CAD build for the part. Positions are in the model's coordinates, mm. A direction names the side the tool comes from. Round coordinates to 2 decimals unless told otherwise and drop trailing zeros. Order: outer loops, then holes, each group sorted by start corner. A loop starts at its lowest first (then second) coordinate and runs counter-clockwise, first axis right, second up. Notation, with made-up numbers: (-7.75, -6.75) -> (1.25, -6.75) arc R19 cw to (1.25, 29.25) -> close; hole circle Ø1 at (-25.75, -40). An arc over 180 degrees is marked (long way). Return JSON: item names as keys, results as strings. Group by question number.
Q1. Which spindle directions (+Z, -Z, +X, -X, +Y, -Y) get a long thin tool onto all of the face, cutting with end or side? Do faces 1 (the cylindrical face through (-10.67, 23.42, 31.62)), 2 (the flat face through (-4, -1, -11.1)), 3 (the flat face through (0, 13, 30.1)). Say none if no direction does.
Q2. Flat gauge pin, fed straight in: pin 1 (2.5 mm diameter, centred on x = -11, z = -34, fed in from +Y). Where does the tip first touch, or does it go through?
Q3. Cut at B-B (x = 11). Write the cut outline in (y, z), then the cut area to 3 significant figures.
Q4. Cut at D-D (z = -34.1). Write the cut outline in (x, y), then the cut area to 3 significant figures.
Q5. Probe line 1 along Z through (x, y) = (-11, 23.2); line 2 along X through (y, z) = (23.7, 34.1); line 3 along Z through (x, y) = (-2.75, 3). List the from-to ranges inside material, lowest first.
Q6. Cut at A-A (y = 20). Write the cut outline in (x, z).
Q7. Cut at C-C (z = 7). Write the cut outline in (x, y) (3 decimals), then the cut area to 3 significant figures.
Q8. Mould opens along X. For faces 4 (the flat face through (-15, -4, 1)), 5 (the cylindrical face through (11.33, 23.42, 31.62)), 6 (the flat face through (0, 8, -38.1)) say: +X half, -X half, draft (parallel to the pull), parting line (faces both ways), or undercut.
from build123d import *

# Parameters (mm, degrees)
SKETCH1_W                       = 30
SKETCH1_H                       = 76.2
BOSS_EXTRUDE1_DEPTH             = 10
SKETCH2_W                       = 22.6
SKETCH2_H                       = 22.2
CUT_EXTRUDE2_DEPTH              = 2.335
SKETCH3_W                       = 30
SKETCH3_H                       = 8
BOSS_EXTRUDE2_DEPTH             = 26
F_5_0MM_DOWEL_HOLE1_D           = 5
F_5_0MM_DOWEL_HOLE1_DEPTH       = 4.6
F_5_0MM_DOWEL_HOLE1_CSINK_D     = 6
F_5_0MM_DOWEL_HOLE1_CSINK_ANGLE = 90
FILLET1_R                       = 1


with BuildPart() as part:
    # Sketch1 → Boss-Extrude1 (new body)
    with BuildSketch(Plane(origin=(0, 0, 0), x_dir=(1, 0, 0), z_dir=(0, 1, 0))):
        Rectangle(SKETCH1_W, SKETCH1_H)
    extrude(amount=-BOSS_EXTRUDE1_DEPTH)

    # Sketch2 → Cut-Extrude2 (cut)
    with BuildSketch(Plane(origin=(0, 0, 0), x_dir=(1, 0, 0), z_dir=(0, 1, 0))):
        with Locations((-3.7, 0)):
            Rectangle(SKETCH2_W, SKETCH2_H)
    extrude(amount=-CUT_EXTRUDE2_DEPTH, mode=Mode.SUBTRACT)

    # Sketch3 → Boss-Extrude2 (add)
    with BuildSketch(Plane(origin=(0, 0, 0), x_dir=(1, 0, 0), z_dir=(0, 1, 0))):
        with Locations((0, 34.1)):
            Rectangle(SKETCH3_W, SKETCH3_H)
        with Locations((0, -34.1)):
            Rectangle(SKETCH3_W, SKETCH3_H)
    extrude(amount=BOSS_EXTRUDE2_DEPTH)

    # Ø5.0mm Dowel Hole1
    with Locations(Plane(origin=(0, 26, 0), x_dir=(1, 0, 0), z_dir=(0, 1, 0))):
        with Locations((-11, 34.1), (11, 34.1), (11, -34.1), (-11, -34.1)):
            CounterSinkHole(F_5_0MM_DOWEL_HOLE1_D / 2, F_5_0MM_DOWEL_HOLE1_CSINK_D / 2, depth=F_5_0MM_DOWEL_HOLE1_DEPTH, counter_sink_angle=F_5_0MM_DOWEL_HOLE1_CSINK_ANGLE)

    # Fillet1
    fillet1_edges = [part.edges().sort_by_distance(p)[0] for p in [
        (-15, 13, -30.1),
        (15, 13, -30.1),
        (-15, 13, 30.1),
        (15, 13, 30.1),
        (-15, 8, -38.1),
        (15, 8, -38.1),
        (15, 8, 38.1),
        (-15, 8, 38.1),
    ]]
    fillet(fillet1_edges, radius=FILLET1_R)


solid = part.part
Solution:
{
 "1": {"face 1": "+Y", "face 2": "-X, +Y", "face 3": "+X, -X, +Y"},
 "2": {"pin 1": "stops at y = 21.4"},
 "3": {"outline": "(-10, -38.1) -> (26, -38.1) -> (26, -37.1) -> (25.5, -36.6) -> (21.4, -36.6) -> (21.4, -31.6) -> (25.5, -31.6) -> (26, -31.1) -> (26, -30.1) -> (0, -30.1) -> (0, 30.1) -> (26, 30.1) -> (26, 31.1) -> (25.5, 31.6) -> (21.4, 31.6) -> (21.4, 36.6) -> (25.5, 36.6) -> (26, 37.1) -> (26, 38.1) -> (-10, 38.1) -> close", "area": "1,130 mm²"},
 "4": {"outline": "(-15, -10) -> (15, -10) -> (15, 26) -> (14, 26) -> (13.5, 25.5) -> (13.5, 21.4) -> (8.5, 21.4) -> (8.5, 25.5) -> (8, 26) -> (-8, 26) -> (-8.5, 25.5) -> (-8.5, 21.4) -> (-13.5, 21.4) -> (-13.5, 25.5) -> (-14, 26) -> (-15, 26) -> close", "area": "1,030 mm²"},
 "5": {"line 1": "z = -38.1 to -36.6, -31.6 to -30.1, 30.1 to 31.6, 36.6 to 38.1", "line 2": "x = -15 to -13.5, -8.5 to 8.5, 13.5 to 15", "line 3": "z = -38.1 to -30.1, 30.1 to 38.1"},
 "6": {"outline": "(-15, -37.1) arc R1 ccw to (-14, -38.1) -> (14, -38.1) arc R1 ccw to (15, -37.1) -> (15, -31.1) arc R1 ccw to (14, -30.1) -> (-14, -30.1) arc R1 ccw to (-15, -31.1) -> close; (-15, 31.1) arc R1 ccw to (-14, 30.1) -> (14, 30.1) arc R1 ccw to (15, 31.1) -> (15, 37.1) arc R1 ccw to (14, 38.1) -> (-14, 38.1) arc R1 ccw to (-15, 37.1) -> close"},
 "7": {"outline": "(-15, -10) -> (15, -10) -> (15, 0) -> (7.6, 0) -> (7.6, -2.335) -> (-15, -2.335) -> close", "area": "247 mm²"},
 "8": {"face 4": "-X half", "face 5": "undercut", "face 6": "draft"}
}
